Design review of the part built by this model. Coordinates are the model's own, in mm. Face numbers are marked on the shaded views. A direction names the side the tool comes from. Give positions to 0.01 mm unless a question says otherwise; leave off trailing zeros. Write each loop counter-clockwise with the first axis right and the second up, starting at its lowest first coordinate (ties: lowest second). Pieces come first, ordered by that corner, then holes.
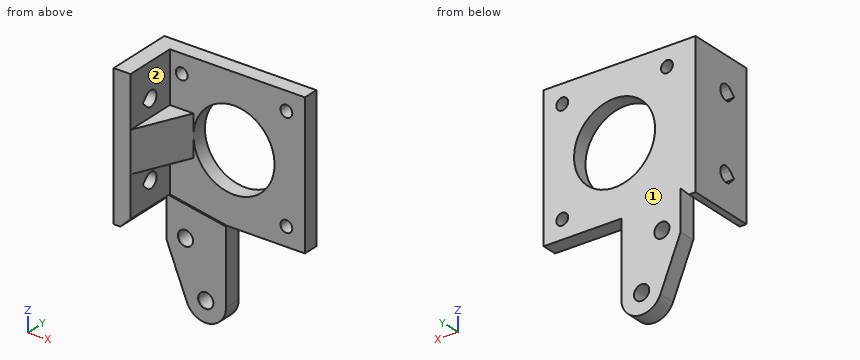
```python
from build123d import *

# Parameters (mm, degrees)
BOSS_EXTRUDE1_DEPTH = 21
CUT_EXTRUDE1_REACH  = 55.535
SKETCH2_R           = 12
SKETCH2_R_2         = 1.75
BOSS_EXTRUDE2_DEPTH = 6
CUT_EXTRUDE2_DEPTH  = 50.406477308
SKETCH5_R           = 2.25
BOSS_EXTRUDE3_DEPTH = 4.5
CHAMFER1_SIZE       = 3
SKETCH6_R           = 2.25
BOSS_EXTRUDE4_DEPTH = 0.5


with BuildPart() as part:
    # Sketch1 → Boss-Extrude1 (new, symmetric)
    with BuildSketch(Plane.XY):
        Polygon((0, 0), (45, 0), (45, -4.5), (5, -4.5), (5, -20), (0, -20), align=None)
    extrude(amount=BOSS_EXTRUDE1_DEPTH, both=True)

    # Sketch2 → Cut-Extrude1 (cut, up to next)
    with BuildSketch(Plane(origin=(0, 0, 0), x_dir=(1, 0, 0), z_dir=(0, 1, 0)), mode=Mode.PRIVATE) as cut_extrude1_sk1:
        with Locations(Location((24, 0, 0), (0, 0, 270))):
            Circle(SKETCH2_R)
    cut_extrude1_tool1 = extrude(cut_extrude1_sk1.sketch, amount=-CUT_EXTRUDE1_REACH, mode=Mode.PRIVATE) & part.part
    # Sketch2 → Cut-Extrude1 (cut, up to next)
    with BuildSketch(Plane(origin=(0, 0, 0), x_dir=(1, 0, 0), z_dir=(0, 1, 0)), mode=Mode.PRIVATE) as cut_extrude1_sk2:
        with Locations(Location((39.5, 15.5, 0), (0, 0, 270))):
            Circle(SKETCH2_R_2)
    cut_extrude1_tool2 = extrude(cut_extrude1_sk2.sketch, amount=-CUT_EXTRUDE1_REACH, mode=Mode.PRIVATE) & part.part
    # Sketch2 → Cut-Extrude1 (cut, up to next)
    with BuildSketch(Plane(origin=(0, 0, 0), x_dir=(1, 0, 0), z_dir=(0, 1, 0)), mode=Mode.PRIVATE) as cut_extrude1_sk3:
        with Locations(Location((8.5, -15.5, 0), (0, 0, 270))):
            Circle(SKETCH2_R_2)
    cut_extrude1_tool3 = extrude(cut_extrude1_sk3.sketch, amount=-CUT_EXTRUDE1_REACH, mode=Mode.PRIVATE) & part.part
    # Sketch2 → Cut-Extrude1 (cut, up to next)
    with BuildSketch(Plane(origin=(0, 0, 0), x_dir=(1, 0, 0), z_dir=(0, 1, 0)), mode=Mode.PRIVATE) as cut_extrude1_sk4:
        with Locations(Location((39.5, -15.5, 0), (0, 0, 270))):
            Circle(SKETCH2_R_2)
    cut_extrude1_tool4 = extrude(cut_extrude1_sk4.sketch, amount=-CUT_EXTRUDE1_REACH, mode=Mode.PRIVATE) & part.part
    add(cut_extrude1_tool1.solids().sort_by_distance((24, 0, 0))[0], mode=Mode.SUBTRACT)
    add(cut_extrude1_tool2.solids().sort_by_distance((39.5, 0, -15.5))[0], mode=Mode.SUBTRACT)
    add(cut_extrude1_tool3.solids().sort_by_distance((8.5, 0, 15.5))[0], mode=Mode.SUBTRACT)
    add(cut_extrude1_tool4.solids().sort_by_distance((39.5, 0, 15.5))[0], mode=Mode.SUBTRACT)

    # Sketch3 → Boss-Extrude2 (add, symmetric)
    with BuildSketch(Plane.XY):
        Polygon((5, -20), (12, -4.5), (5, -4.5), align=None)
    extrude(amount=BOSS_EXTRUDE2_DEPTH, both=True)

    # Sketch4 → Cut-Extrude2 (cut, through all)
    with BuildSketch(Plane(origin=(5, 0, 0), x_dir=(0, 0, -1), z_dir=(1, 0, 0))):
        with BuildLine():
            Line((9.409009742, -13.590990258), (11, -15.181980515))
            Line((11, -15.181980515), (12.590990258, -13.590990258))
            ThreePointArc((12.590990258, -13.590990258), (11, -9.75), (9.409009742, -13.590990258))
        make_face()
        with BuildLine():
            Line((-12.590990258, -13.590990258), (-11, -15.181980515))
            Line((-11, -15.181980515), (-9.409009742, -13.590990258))
            ThreePointArc((-9.409009742, -13.590990258), (-11, -9.75), (-12.590990258, -13.590990258))
        make_face()
    extrude(amount=-CUT_EXTRUDE2_DEPTH, mode=Mode.SUBTRACT)

    # Sketch5 → Boss-Extrude3 (add)
    with BuildSketch(Plane(origin=(0, 0, 0), x_dir=(1, 0, 0), z_dir=(0, 1, 0))):
        with BuildLine():
            Line((4.437851135, 30.25), (10.437851135, 45.082396974))
            ThreePointArc((10.437851135, 45.082396974), (17.146103575, 48.721917039), (22, 42.832396974))
            Line((22, 42.832396974), (22, 21))
            Line((22, 21), (4.437851135, 21))
            Line((4.437851135, 21), (4.437851135, 30.25))
        make_face()
        with Locations(Location((10, 28, 0), (0, 0, 270))):
            Circle(SKETCH5_R, mode=Mode.SUBTRACT)
        with Locations(Location((16, 42.832396974, 0), (0, 0, 270))):
            Circle(SKETCH5_R, mode=Mode.SUBTRACT)
    extrude(amount=-BOSS_EXTRUDE3_DEPTH)

    # Chamfer1
    chamfer1_edges = [part.edges().sort_by_distance(p)[0] for p in [
        (5, -12.25, -21),
    ]]
    chamfer(chamfer1_edges, length=CHAMFER1_SIZE)

    # Sketch6 → Boss-Extrude4 (add)
    with BuildSketch(Plane.XZ.offset(4.5)):
        with BuildLine():
            Line((5, -18), (22, -21))
            Line((22, -21), (22, -42.832396974))
            ThreePointArc((22, -42.832396974), (17.146103575, -48.721917039), (10.437851135, -45.082396974))
            Line((10.437851135, -45.082396974), (4.437851135, -30.25))
            Line((4.437851135, -30.25), (4.437851135, -18.562148865))
            Line((4.437851135, -18.562148865), (5, -18))
        make_face()
        with Locations(Location((10, -28, 0), (0, 0, 90))):
            Circle(SKETCH6_R, mode=Mode.SUBTRACT)
        with Locations(Location((16, -42.832396974, 0), (0, 0, 90))):
            Circle(SKETCH6_R, mode=Mode.SUBTRACT)
    extrude(amount=BOSS_EXTRUDE4_DEPTH)


solid = part.part
```
(1) Consider section B-B, the plane x = 39.5. Give the boundary of the cut face in (y, z).
Resolved:
outline: (-4.5, -21) - (0, -21) - (0, -17.25) - (-4.5, -17.25) - close; (-4.5, -13.75) - (0, -13.75) - (0, 13.75) - (-4.5, 13.75) - close; (-4.5, 17.25) - (0, 17.25) - (0, 21) - (-4.5, 21) - close
(2) Tool access review of the marked faces 1 and 2: name each direction out of +Z, -Z, +X, -X, +Y, -Y from which nothing blocks a thin tool from reaching the whole face with its end or side.
Resolved:
face 1: +Z, -Z, +X, -X, +Y
face 2: +Z, +X, -Y
(3) Consider section A-A, the plane z = 15.5. Give the boundary of the cut face in (x, y).
Resolved:
outline: (0, -20) - (5, -20) - (5, -4.5) - (6.75, -4.5) - (6.75, 0) - (0, 0) - close; (10.25, -4.5) - (37.75, -4.5) - (37.75, 0) - (10.25, 0) - close; (41.25, -4.5) - (45, -4.5) - (45, 0) - (41.25, 0) - close
(4) Clearance check with flat-ended pins moving along their axes: P1, Ø5, axis at y = -10.5, z = 12, coming from the +X side; P2, Ø5.5, axis at y = -1.5, z = -37.5, coming from the +X side; P3, Ø2, axis at x = 1, y = -5.5, coming from the -Z side. State where each tip first meets the part, or that it passes through.
Resolved:
P1: stops at x = 5
P2: stops at x = 22
P3: stops at z = -21
(5) To check wall thickness, follow L1, parallel to Z at x = 1.4, y = -12; L2, parallel to Z at x = 10, y = -4.9; L3, parallel to Z at x = 24, y = -3.2. State the ranges of each line that lie inside material, in increasing order.
Resolved:
L1: z = -21 to -13.25, -8.75 to 8.75, 13.25 to 21
L2: z = -44 to -30.25, -25.75 to -18.88, -6 to 6
L3: z = -21 to -12, 12 to 21
(6) Consider section D-D, the plane z = -15.5. Give the boundary of the cut face in (x, y), then the cut area to 3 significant figures.
Resolved:
outline: (0, -20) - (5, -20) - (5, -4.5) - (37.75, -4.5) - (37.75, 0) - (0, 0) - close; (41.25, -4.5) - (45, -4.5) - (45, 0) - (41.25, 0) - close
area: 264 mm2
(7) Consider section C-C, the plane y = -12. Give the boundary of the cut face in (x, z).
Resolved:
outline: (0, -21) - (2, -21) - (5, -18) - (5, -13.25) - (0, -13.25) - close; (0, -8.75) - (5, -8.75) - (5, -6) - (8.61, -6) - (8.61, 6) - (5, 6) - (5, 8.75) - (0, 8.75) - close; (0, 13.25) - (5, 13.25) - (5, 21) - (0, 21) - close
